Verification items for the finished model (mm, model axes). Face numbers are marked on the shaded views. A direction names the side the tool comes from. Round coordinates to 2 decimals unless told otherwise and drop trailing zeros. Write each loop counter-clockwise with the first axis right and the second up, starting at its lowest first coordinate (ties: lowest second). Pieces come first, ordered by that corner, then holes. Notation, with made-up numbers: (0, 29) - (55, 29) arc R33 cw to (55, 68) - close; hole circle Ø7 at (38.25, -18). An arc over 180 degrees is marked (long way). Answer as a JSON object with one key per item and string values. Group by question number.
1) Thickness scan on line 1 (X direction, y = -36, z = 4); line 2 (Z direction, x = 4, y = -12); line 3 (Z direction, x = 2.75, y = -36). Record the ranges inside material, lowest first.
2) Section check D-D (y = -26). Enter the section's corners in (x, z).
3) Section check C-C (z = 40.5). Enter the section's corners in (x, y).
4) Mould release check, pull along X, two halves, no side actions. Record for the marked faces 4, 5 and 6: +X half, -X half, draft (parallel to the pull), parting line (faces both ways), or undercut.
5) Go/stop test with flat-tipped pins: pin 1 Ø6 at (y, z) = (-22, 35.5) entering from +X; pin 2 Ø9.5 at (x, y) = (53.23, -12) entering from -Z; pin 3 Ø17.5 at (y, z) = (-20, 25) entering from +X; pin 4 Ø5 at (x, y) = (37, -31) entering from +Z. Record where each tip stops, or that it passes through.
6) Section check A-A (y = -12). Enter the section's corners in (x, z), then the cut area to 4 significant figures.
7) Section check B-B (x = 35). Enter the section's corners in (y, z).
8) Set-up check for the marked faces 1, 2 and 3: record each of +Z, -Z, +X, -X, +Y, -Y from which the full face is reachable in a straight line by a thin tool's end or side.
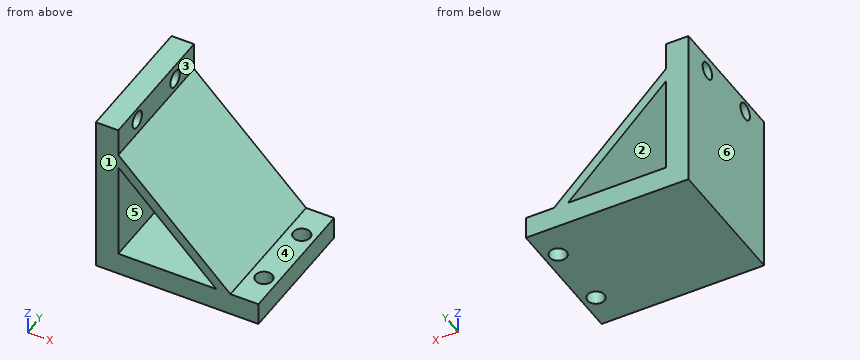
```python
from build123d import *

# Parameters (mm, degrees)
F1_DEPTH = 48
F2_R     = 3
F3_DEPTH = 25
F4_R     = 3
F5_DEPTH = 25


with BuildPart() as f1:
    # F0 (on Front) → F1 (new body)
    with BuildSketch(Plane.XZ):
        Polygon((0, 8), (0, 0), (58, 0), (58, 8), (48, 8), (43, 8), (8, 8), align=None)
        Polygon((43, 8), (48, 8), (8, 48), (8, 43), align=None)
        Polygon((0, 58), (0, 8), (8, 8), (8, 43), (8, 48), (8, 58), align=None)
    extrude(amount=F1_DEPTH)

    # F2 (on Right) → F3 (cut)
    with BuildSketch(Plane.YZ):
        with Locations((-36, 53.59669)):
            Circle(F2_R)
        with Locations((-12, 52.631229)):
            Circle(F2_R)
    extrude(amount=F3_DEPTH, mode=Mode.SUBTRACT)

    # F4 (on Top) → F5 (cut)
    with BuildSketch(Plane.XY):
        with Locations((53.227946, -36)):
            Circle(F4_R)
        with Locations((53.227946, -12)):
            Circle(F4_R)
    extrude(amount=F5_DEPTH, mode=Mode.SUBTRACT)


solid = f1.part
```
Returned:
{
 "1": {"line 1": "0 to 50.23, 56.23 to 58", "line 2": "0 to 49.63, 55.63 to 58", "line 3": "0 to 50.6, 56.6 to 58"},
 "2": {"outline": "(0, 0) - (58, 0) - (58, 8) - (48, 8) - (8, 48) - (8, 58) - (0, 58) - close; hole (8, 8) - (43, 8) - (8, 43) - close"},
 "3": {"outline": "(0, -48) - (8, -48) - (8, 0) - (0, 0) - close; (10.5, -48) - (15.5, -48) - (15.5, 0) - (10.5, 0) - close"},
 "4": {"face 4": "draft", "face 5": "undercut", "face 6": "-X half"},
 "5": {"pin 1": "x = 23.5", "pin 2": "z = 0", "pin 3": "x = 39.75", "pin 4": "z = 21.5"},
 "6": {"outline": "(0, 0) - (50.23, 0) - (50.23, 8) - (48, 8) - (8, 48) - (8, 49.63) - (0, 49.63) - close; (0, 55.63) - (8, 55.63) - (8, 58) - (0, 58) - close; (56.23, 0) - (58, 0) - (58, 8) - (56.23, 8) - close; hole (8, 8) - (43, 8) - (8, 43) - close", "area": "955.5 mm2"},
 "7": {"outline": "(-48, 0) - (0, 0) - (0, 8) - (-48, 8) - close; (-48, 16) - (0, 16) - (0, 21) - (-48, 21) - close"},
 "8": {"face 1": "+Z, -Z, +X, -X, -Y", "face 2": "+Y, -Y", "face 3": "+Z, +X, +Y, -Y"}
}
